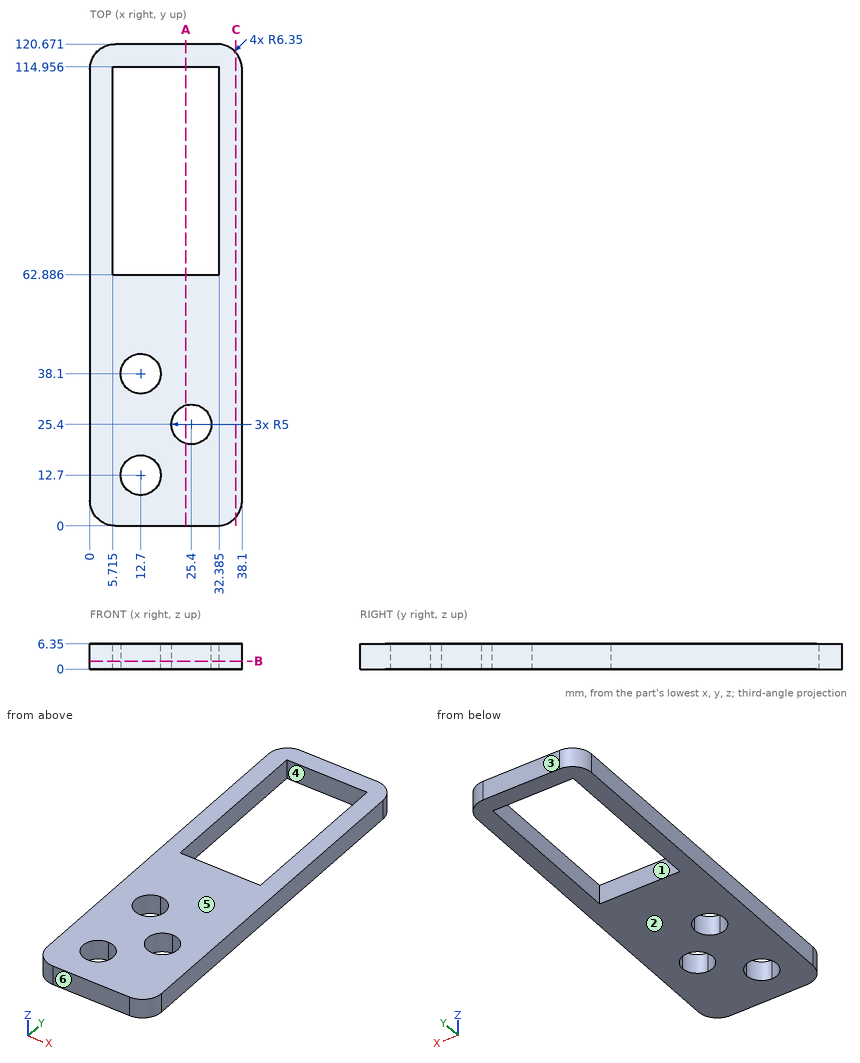
Input: dimensioned drawing with shaded views. Units: mm. Origin: part minimum x, y, z. A direction names the side the tool comes from. Round coordinates to 2 decimals unless told otherwise and drop trailing zeros. Order: outer loops, then holes, each group sorted by start corner. A loop starts at its lowest first (then second) coordinate and runs counter-clockwise, first axis right, second up.
1. Material intervals for line 1 (Y direction, x = 13, z = 4.25); line 2 (X direction, y = 104, z = 1.5) (1 decimal); line 3 (Y direction, x = 29, z = 1) (1 decimal), sorted ascending.
The answers:
line 1: y = 0 to 7.71, 17.69 to 33.11, 43.09 to 62.89, 114.96 to 120.67
line 2: x = 0 to 5.7, 32.4 to 38.1
line 3: y = 0 to 21.9, 28.9 to 62.9, 115 to 120.7
2. Set-up query: the marked faces 1 and 2. Return all of +Z, -Z, +X, -X, +Y, -Y with unobstructed straight access to the full face (end or side cutting, diameter ignored); none if empty.
The answers:
face 1: +Z, -Z
face 2: -Z, +X, -X, +Y, -Y
3. Cut plane B-B, the plane z = 2. State how many separate pieces and enclosed holes the cut face has, then the cut area to 3 significant figures.
The answers:
separate pieces: 1
enclosed holes: 4
area: 2,940 mm2
4. Cut plane A-A, the plane x = 24. Output: boundary loops of the cut face in (y, z), then the cut area to 3 significant figures.
The answers:
outline: (0, 0) - (20.6, 0) - (20.6, 6.35) - (0, 6.35) - close; (30.2, 0) - (62.89, 0) - (62.89, 6.35) - (30.2, 6.35) - close; (114.96, 0) - (120.67, 0) - (120.67, 6.35) - (114.96, 6.35) - close
area: 375 mm2
5. Mould query, pull axis Y, two halves, no side actions, for the marked faces 3, 4, 5 and 6. Classes: released by +Y, released by -Y, zero draft, split by the parting line, or undercut.
The answers:
face 3: released by +Y
face 4: undercut
face 5: zero draft
face 6: released by -Y
6. Cut plane C-C, the plane x = 36.5. Output: boundary loops of the cut face in (y, z), then the cut area to 3 significant figures.
The answers:
outline: (2.14, 0) - (118.54, 0) - (118.54, 6.35) - (2.14, 6.35) - close
area: 739 mm2
7. Pin query (flat end, axial travel): P1, Ø3, axis at x = 10, z = 5, coming from the -Y side. Return the tip coordinate at first contact, or that it passes through.
The answers:
P1: stops at y = 0
